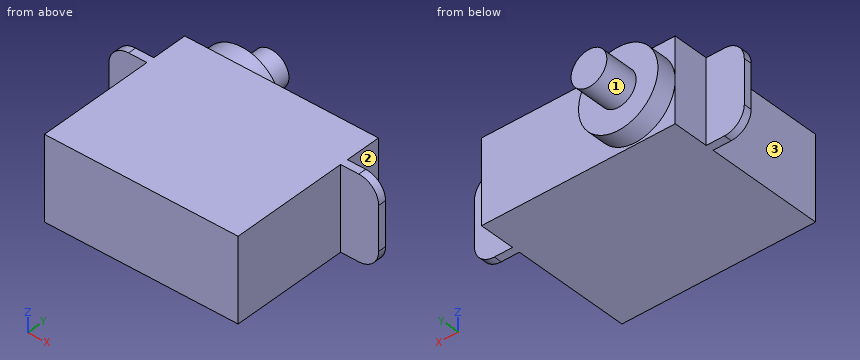
from build123d import *

# Parameters (mm, degrees)
SKETCH1_W           = 19.5
SKETCH1_H           = 8.4
BOSS_EXTRUDE1_DEPTH = 16.3
SKETCH2_R           = 4
BOSS_EXTRUDE2_DEPTH = 2
SKETCH3_W           = 8.4
SKETCH3_H           = 0.8
BOSS_EXTRUDE3_DEPTH = 3.835
FILLET1_R           = 2
FILLET2_R           = 2
SKETCH4_R           = 1.8
BOSS_EXTRUDE4_DEPTH = 3.4


with BuildPart() as part:
    # Sketch1 → Boss-Extrude1 (new body)
    with BuildSketch(Plane(origin=(0, 0, 0), x_dir=(1, 0, 0), z_dir=(0, 1, 0))):
        with Locations((9.75, 4.2)):
            Rectangle(SKETCH1_W, SKETCH1_H)
    extrude(amount=BOSS_EXTRUDE1_DEPTH)

    # Sketch2 → Boss-Extrude2 (add)
    with BuildSketch(Plane(origin=(0, 16.3, 0), x_dir=(1, 0, 0), z_dir=(0, 1, 0))):
        with Locations((4, 4.2)):
            Circle(SKETCH2_R)
    extrude(amount=BOSS_EXTRUDE2_DEPTH)

    # Sketch3 → Boss-Extrude3 (add)
    with BuildSketch(Plane(origin=(19.5, 0, 0), x_dir=(0, 0, -1), z_dir=(1, 0, 0))):
        with Locations((4.2, 12.3)):
            Rectangle(SKETCH3_W, SKETCH3_H)
    boss_extrude3 = extrude(amount=BOSS_EXTRUDE3_DEPTH)

    # Fillet1
    fillet1_edges = [part.edges().sort_by_distance(p)[0] for p in [
        (23.335, 12.3, 0),
        (23.335, 12.3, -8.4),
    ]]
    fillet(fillet1_edges, radius=FILLET1_R)

    # Mirror1: Boss-Extrude3 across plane
    add(boss_extrude3.mirror(Plane(origin=(9.75, 0, 0), x_dir=(0, 0, 1), z_dir=(1, 0, 0))))

    # Fillet2
    fillet2_edges = [part.edges().sort_by_distance(p)[0] for p in [
        (-3.835, 12.3, 0),
        (-3.835, 12.3, -8.4),
    ]]
    fillet(fillet2_edges, radius=FILLET2_R)

    # Sketch4 → Boss-Extrude4 (add)
    with BuildSketch(Plane(origin=(0, 18.3, 0), x_dir=(1, 0, 0), z_dir=(0, 1, 0))):
        with Locations((4, 4.2)):
            Circle(SKETCH4_R)
    extrude(amount=BOSS_EXTRUDE4_DEPTH)


solid = part.part
Check sheet for the modelled part. Datum: model origin and axes. Units: mm. Face numbers are marked on the shaded views. A direction names the side the tool comes from. Round coordinates to 2 decimals unless told otherwise and drop trailing zeros. Loops run counter-clockwise (first coordinate to the right, second up) from the corner with the lowest first, then second, coordinate; pieces in that order, holes last. Notation, with made-up numbers: (9, -36.5) -> (33, -36.5) arc R9 ccw to (33, -32.5) -> close; hole circle Ø9 at (-5.75, 38). An arc over 180 degrees is marked (long way). Put each result on its own line as item: value. Start each with the question number.
1. Scan lines: probe 1 along X at (y, z) = (4.75, -5.25); probe 2 along Y at (x, z) = (18, -5); probe 3 along Y at (x, z) = (2, -3.25). Record each from-to range of solid material in increasing order.
2. Section check A-A (x = 4). Enter the section's corners in (y, z).
3. Section check B-B (z = -3.75). Enter the section's corners in (x, y) (3 decimals), plus the area to 3 significant figures.
4. Section check D-D (x = 1.25). Enter the section's corners in (y, z), plus the area to 3 significant figures.
5. Gauge pin test, flat ends, axial feed: pin 1 (4 mm diameter, centred on y = 6, z = -4, fed in from +X); pin 2 (12 mm diameter, centred on x = 7.5, y = 19, fed in from -Z); pin 3 (2 mm diameter, centred on x = 7, z = -2, fed in from +Y); pin 4 (4 mm diameter, centred on y = 19, z = -1.5, fed in from -X). Record the tip position at first contact, or that the pin passes through.
6. Access from +Z, -Z, +X, -X, +Y, -Y to the whole of each face (thin tool, end or side, straight path). Record for the marked faces 1, 2 and 3.
7. Section check C-C (y = 7). Enter the section's corners in (x, z).
Findings:
1. probe 1: x = 0 to 19.5
1. probe 2: y = 0 to 16.3
1. probe 3: y = 0 to 18.3
2. outline: (0, -8.4) -> (16.3, -8.4) -> (16.3, -8.2) -> (18.3, -8.2) -> (18.3, -6) -> (21.7, -6) -> (21.7, -2.4) -> (18.3, -2.4) -> (18.3, -0.2) -> (16.3, -0.2) -> (16.3, 0) -> (0, 0) -> close
3. outline: (-3.835, 11.9) -> (0, 11.9) -> (0, 0) -> (19.5, 0) -> (19.5, 11.9) -> (23.335, 11.9) -> (23.335, 12.7) -> (19.5, 12.7) -> (19.5, 16.3) -> (7.975, 16.3) -> (7.975, 18.3) -> (5.743, 18.3) -> (5.743, 21.7) -> (2.257, 21.7) -> (2.257, 18.3) -> (0.025, 18.3) -> (0.025, 16.3) -> (0, 16.3) -> (0, 12.7) -> (-3.835, 12.7) -> close
3. area: 352 mm^2
4. outline: (0, -8.4) -> (16.3, -8.4) -> (16.3, -7.1) -> (18.3, -7.1) -> (18.3, -1.3) -> (16.3, -1.3) -> (16.3, 0) -> (0, 0) -> close
4. area: 149 mm^2
5. pin 1: stops at x = 19.5
5. pin 2: stops at z = -8.4
5. pin 3: stops at y = 18.3
5. pin 4: stops at x = 0.09
6. face 1: +Y
6. face 2: +Z, -Z, +X, +Y
6. face 3: +Z, -Z, -X, -Y
7. outline: (0, -8.4) -> (19.5, -8.4) -> (19.5, 0) -> (0, 0) -> close
